Here's the drawing with two shaded views (mm, measured from the low corner). I have some questions. A direction names the side the tool comes from. Give positions to 0.01 mm unless a question says otherwise; leave off trailing zeros. Write each question's results on one line, items separated by ' | '. Start each with the question number.
Q1. If I drill on line 1 along X through (y, z) = (3.05, 19) (1 decimal); line 2 along Z through (x, y) = (44, 2.6) (1 decimal); line 3 along Z through (x, y) = (35, 1.65), over which ranges is the centre line in solid material (lowest first)?
Q2. Which directions (+Z, -Z, +X, -X, +Y, -Y) give clear straight access to the entire face, cutting with the end or side of a thin tool? Please do the marked faces 3 and 4.
Q3. We'd pull the mould along X, two halves only. Please class the marked faces 1 and 2: released by +X, released by -X, zero draft, split by the parting line, or undercut.
Q4. Will these pins go through, and if not, where does the flat tip stop? P1, Ø2.5, axis at x = 6.85, z = 51.25, coming from the +Y side; P2, Ø2.5, axis at y = 3.5, z = 9.5, coming from the -X side; P3, Ø4, axis at x = 40, z = 47, coming from the -Y side; P4, Ø2, axis at y = 2.5, z = 33.5, coming from the -X side.
Q5. If we section it at A-A, the plane y = 3.8: Give the number of separate pieces and of enclosed holes in the cut face, plus the area to 3 significant figures.
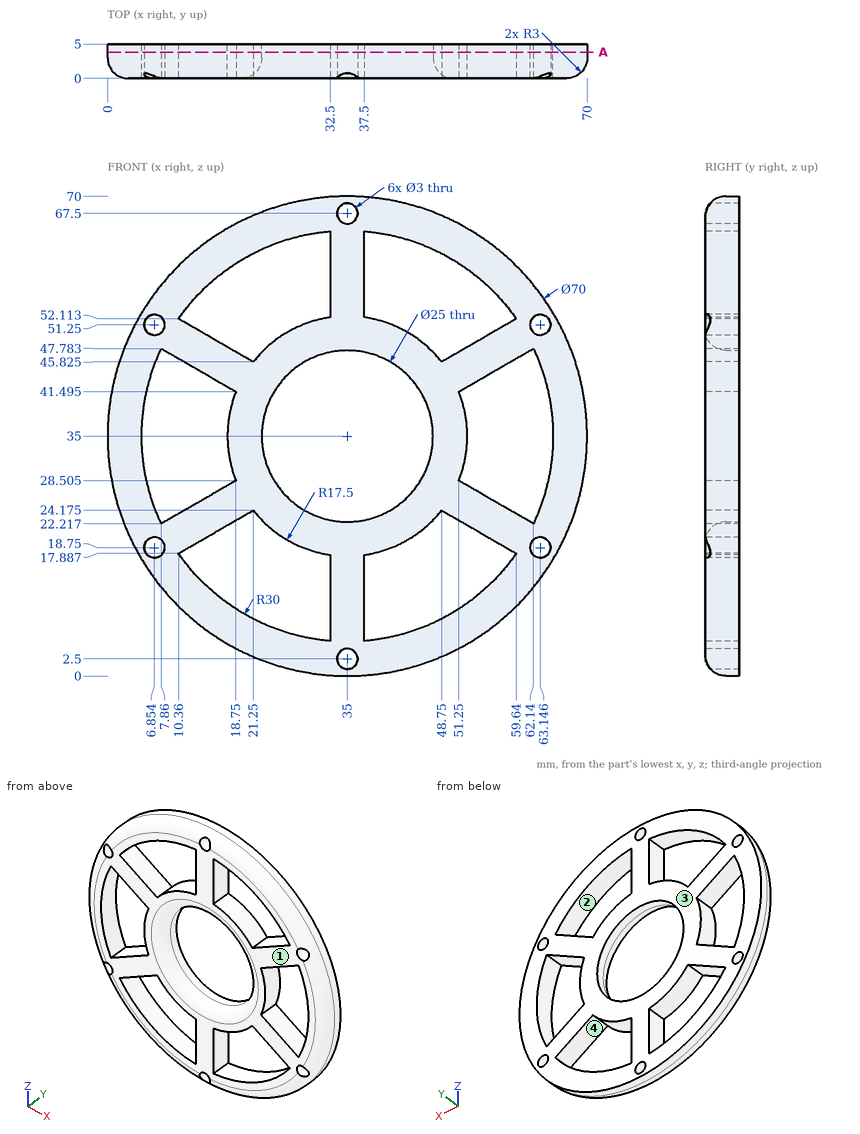
Final values:
1) line 1: x = 3.9 to 5.4, 8.3 to 12.3, 27.9 to 42.1, 57.7 to 61.7, 64.6 to 66.1 | line 2: z = 1.2 to 6.4, 20 to 26.3, 43.7 to 50, 63.6 to 68.8 | line 3: z = 0.32 to 1, 4 to 22.18, 47.82 to 66, 69 to 69.68
2) face 3: +Z, -Z, +X, -X, +Y | face 4: +Y, -Y
3) face 1: zero draft | face 2: undercut
4) P1: passes through | P2: stops at x = 9.76 | P3: stops at y = 0.04 | P4: stops at x = 0.01
5) separate pieces: 1 | enclosed holes: 13 | area: 1,830 mm²
